The listing builds one solid part. Answer for the finished solid, in the listing's coordinates (mm). Give positions to 0.01 mm unless a question says otherwise; leave off trailing zeros. Write each loop counter-clockwise with the first axis right and the second up, starting at its lowest first coordinate (ties: lowest second). Pieces come first, ordered by that corner, then holes. Notation, with made-up numbers: M -9.75,58 L 41.25,58 A27 cw 41.25,81 Z; hole C -17.5,-19 d3. An arc over 180 degrees is marked long. Answer as a JSON object with one key per item and string values.
```python
from build123d import *

# Parameters (mm, degrees)
SKETCH1_W           = 100
SKETCH1_H           = 100
BOSS_EXTRUDE1_DEPTH = 40
SKETCH2_R           = 7.5
BOSS_EXTRUDE2_DEPTH = 10
BOSS_EXTRUDE3_START = 7
SKETCH2_4_R         = 10.5
SKETCH2_4_R_2       = 7.5
BOSS_EXTRUDE3_DEPTH = 10
CHAMFER1_SIZE       = 1
CHAMFER2_SIZE       = 5
FILLET1_R           = 5


# Some blends are built 0.0001 mm under size
with BuildPart() as part:
    # Sketch1 → Boss-Extrude1 (new body)
    with BuildSketch(Plane(origin=(0, 0, 0), x_dir=(1, 0, 0), z_dir=(0, 1, 0))):
        Rectangle(SKETCH1_W, SKETCH1_H)
    extrude(amount=BOSS_EXTRUDE1_DEPTH)

    # Sketch2 → Boss-Extrude2 (add)
    with BuildSketch(Plane(origin=(0, 40, 0), x_dir=(1, 0, 0), z_dir=(0, 1, 0))):
        with Locations(Location((0, -37.5, 0), (0, 0, 90))):
            Circle(SKETCH2_R)
        with Locations(Location((0, -12.5, 0), (0, 0, 90))):
            Circle(SKETCH2_R)
        with Locations(Location((0, 12.5, 0), (0, 0, 90))):
            Circle(SKETCH2_R)
        with Locations(Location((0, 37.5, 0), (0, 0, 90))):
            Circle(SKETCH2_R)
    extrude(amount=BOSS_EXTRUDE2_DEPTH)

    # Sketch2<4> → Boss-Extrude3 (add)
    # profile 1 of 4: a face of its own
    with BuildSketch(Plane(origin=(0, 40, 0), x_dir=(1, 0, 0), z_dir=(0, 1, 0)).offset(BOSS_EXTRUDE3_START)):
        with Locations(Location((0, -37.5, 0), (0, 0, 270))):
            Circle(SKETCH2_4_R)
        with Locations(Location((0, -37.5, 0), (0, 0, 90))):
            Circle(SKETCH2_4_R_2, mode=Mode.SUBTRACT)
    # profile 2 of 4: a face of its own
    with BuildSketch(Plane(origin=(0, 40, 0), x_dir=(1, 0, 0), z_dir=(0, 1, 0)).offset(BOSS_EXTRUDE3_START)):
        with Locations(Location((0, -12.5, 0), (0, 0, 270))):
            Circle(SKETCH2_4_R)
        with Locations(Location((0, -12.5, 0), (0, 0, 90))):
            Circle(SKETCH2_4_R_2, mode=Mode.SUBTRACT)
    # profile 3 of 4: a face of its own
    with BuildSketch(Plane(origin=(0, 40, 0), x_dir=(1, 0, 0), z_dir=(0, 1, 0)).offset(BOSS_EXTRUDE3_START)):
        with Locations(Location((0, 12.5, 0), (0, 0, 270))):
            Circle(SKETCH2_4_R)
        with Locations(Location((0, 12.5, 0), (0, 0, 90))):
            Circle(SKETCH2_4_R_2, mode=Mode.SUBTRACT)
    # profile 4 of 4: a face of its own
    with BuildSketch(Plane(origin=(0, 40, 0), x_dir=(1, 0, 0), z_dir=(0, 1, 0)).offset(BOSS_EXTRUDE3_START)):
        with Locations(Location((0, 37.5, 0), (0, 0, 270))):
            Circle(SKETCH2_4_R)
        with Locations(Location((0, 37.5, 0), (0, 0, 90))):
            Circle(SKETCH2_4_R_2, mode=Mode.SUBTRACT)
    extrude(amount=BOSS_EXTRUDE3_DEPTH)

    # Chamfer1
    chamfer1_edges = [part.edges().sort_by_distance(p)[0] for p in [
        (0, 47, 45),
        (0, 47, 20),
        (0, 47, -5),
        (0, 47, -30),
    ]]
    chamfer(chamfer1_edges, length=CHAMFER1_SIZE)

    # Chamfer2
    # the kernel refuses this chamfer: 5 mm, written as the material it takes off along each edge
    with BuildSketch(Plane(origin=(0, 57, -37.5), x_dir=(0, 0, 1), z_dir=(-1, 0, 0))) as chamfer2_piece_1:
        Polygon((10.5, -CHAMFER2_SIZE), (10.5 - CHAMFER2_SIZE, 0), (10.5, 0), align=None)
    revolve(axis=Axis((0, 57, -37.5), (0, 1, 0)), mode=Mode.SUBTRACT)
    with BuildSketch(Plane(origin=(0, 57, -12.5), x_dir=(0, 0, 1), z_dir=(-1, 0, 0))) as chamfer2_piece_2:
        Polygon((10.5, -CHAMFER2_SIZE), (10.5 - CHAMFER2_SIZE, 0), (10.5, 0), align=None)
    revolve(axis=Axis((0, 57, -12.5), (0, 1, 0)), mode=Mode.SUBTRACT)
    with BuildSketch(Plane(origin=(0, 57, 12.5), x_dir=(0, 0, 1), z_dir=(-1, 0, 0))) as chamfer2_piece_3:
        Polygon((10.5, -CHAMFER2_SIZE), (10.5 - CHAMFER2_SIZE, 0), (10.5, 0), align=None)
    revolve(axis=Axis((0, 57, 12.5), (0, 1, 0)), mode=Mode.SUBTRACT)
    with BuildSketch(Plane(origin=(0, 57, 37.5), x_dir=(0, 0, 1), z_dir=(-1, 0, 0))) as chamfer2_piece_4:
        Polygon((10.5, -CHAMFER2_SIZE), (10.5 - CHAMFER2_SIZE, 0), (10.5, 0), align=None)
    revolve(axis=Axis((0, 57, 37.5), (0, 1, 0)), mode=Mode.SUBTRACT)

    # Fillet1
    fillet1_edges = [part.edges().sort_by_distance(p)[0] for p in [
        (-50, 40, 0),
        (0, 40, 50),
        (50, 40, 0),
        (0, 0, 50),
        (-50, 0, 0),
        (0, 0, -50),
        (50, 0, 0),
        (50, 20, 50),
        (-50, 20, 50),
        (-50, 20, -50),
        (50, 20, -50),
        (0, 40, -50),
    ]]
    fillet(fillet1_edges, radius=FILLET1_R - 0.0001)  # a hair under: the kernel refuses the full size


solid = part.part
```
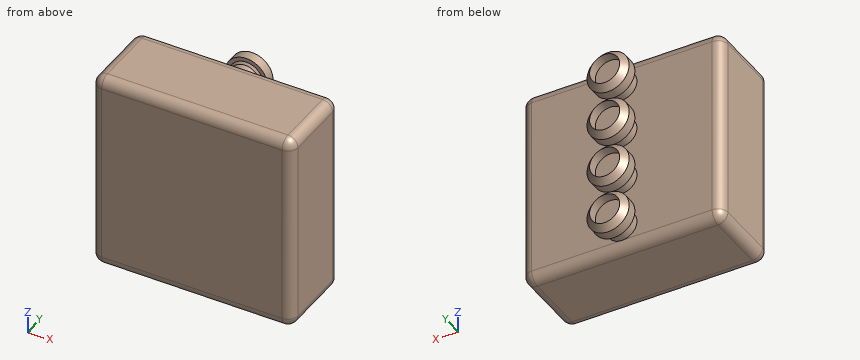
1. Flat-ended cylindrical pins translate along their axes: pin 1 (13.5 mm diameter, centred on x = 0, z = 12.5, fed in from +Y); pin 2 (5 mm diameter, centred on x = 32, z = -10.5, fed in from +Y); pin 3 (16.5 mm diameter, centred on x = -3.5, z = -37.5, fed in from +Y); pin 4 (4 mm diameter, centred on x = 11, z = -38.5, fed in from +Y). Find the tip coordinate at first contact, or state that the pin passes through.
Verdict:
{"pin 1": "stops at y = 50", "pin 2": "stops at y = 40", "pin 3": "stops at y = 55", "pin 4": "stops at y = 53.45"}
2. Consider line 1 along X through (y, z) = (52, 37); line 2 along Y through (x, z) = (3, 42.5); line 3 along Y through (x, z) = (23.5, 24.5). Determine where each line is inside the solid, lowest interval first.
Verdict:
{"line 1": "x = -10.49 to -7.48, 7.48 to 10.49", "line 2": "y = 0 to 50", "line 3": "y = 0 to 40"}
3. A cutting plane is placed at B-B, the plane z = 37.5. Give the vertices of the cut face in (x, y).
Verdict:
{"outline": "M -50,5 A5 ccw -45,0 L 45,0 A5 ccw 50,5 L 50,35 A5 ccw 45,40 L 7.5,40 L 7.5,46 L 8.5,47 L 10.5,47 L 10.5,52 L 7.5,55 L 7.5,50 L -7.5,50 L -7.5,55 L -10.5,52 L -10.5,47 L -8.5,47 L -7.5,46 L -7.5,40 L -45,40 A5 ccw -50,35 Z"}
4. A cutting plane is placed at A-A, the plane x = 34. Give the vertices of the cut face in (y, z), plus the area to 3 significant figures.
Verdict:
{"outline": "M 0,-45 A5 ccw 5,-50 L 35,-50 A5 ccw 40,-45 L 40,45 A5 ccw 35,50 L 5,50 A5 ccw 0,45 Z", "area": "3,980 mm2"}
